Here's how the part is built. I have some questions about the finished solid (model axes, mm). Round coordinates to 2 decimals unless told otherwise and drop trailing zeros. Write each loop counter-clockwise with the first axis right and the second up, starting at its lowest first coordinate (ties: lowest second). Pieces come first, ordered by that corner, then holes. Notation, with made-up numbers: (-16, 29.25) -> (-2, 29.25) arc R15 cw to (-2, 47.25) -> close; hole circle Ø4 at (55, -39). An arc over 180 degrees is marked (long way). Answer in a Markdown table with one row per item.
Autodesk Inventor part; units mm, degrees
ref_plane "YZ Plane" through (0, 0, 0) normal (1, 0, 0) x (0, 1, 0)
ref_plane "XZ Plane" through (0, 0, 0) normal (0, 1, 0) x (-1, 0, 0)
ref_plane "XY Plane" through (0, 0, 0) normal (0, 0, 1) x (1, 0, 0)
sketch "スケッチ1" plane through (0, 0, 0) normal (0, 0, 1) x (1, 0, 0)
  circle A0 centre (0, 0) radius 2
  dimension "d0" = 4
extrude "押し出し1" add sketch "スケッチ1" along normal mid plane 48
chamfer "面取り1" distance 0.1 angle 45 2 edges at (-2, 0, 24) (-2, 0, -24)
sketch "スケッチ2" plane through (0, 0, 0) normal (0, 1, 0) x (-1, 0, 0)
  line L0 (0, 0) -> (3.4806, 0) construction
  line L1 (0, 0) -> (0, -21.75) construction
  circle A0 centre (0, -21.75) radius 0.75
  circle A1 centre (0, 21.75) radius 0.75
  line L2 (2.6688, -21) -> (-4.3603, -21) construction
  dimension "d6" = 1.5
  dimension "d11" = 42
extrude "押し出し2" cut sketch "スケッチ2" along normal through all both and the other way through all
properties part number "COXA_ROLL_SHAFT_D4"
1) I want a section at A-A, the plane x = 0. List the corners of the cut face in (y, z) for me.
Response:
| item | result |
|---|---|
| outline | (-2, -23.9) -> (-1.9, -24) -> (1.9, -24) -> (2, -23.9) -> (2, -22.5) -> (-2, -22.5) -> close; (-2, -21) -> (2, -21) -> (2, 21) -> (-2, 21) -> close; (-2, 22.5) -> (2, 22.5) -> (2, 23.9) -> (1.9, 24) -> (-1.9, 24) -> (-2, 23.9) -> close |
2) I want a section at C-C, the plane z = -21.75. List the corners of the cut face in (x, y) for me.
Response:
| item | result |
|---|---|
| outline | (-0.75, -1.85) -> (-0.75, 1.85) arc R2 ccw to start; (0.75, -1.85) arc R2 ccw to (0.75, 1.85) -> close |
3) I need wall thicknesses on line 1 (Z direction, x = 0, y = 1.2); line 2 (X direction, y = 0.2, z = -21.75); line 3 (X direction, y = -0.1, z = -12). Which ranges of each line are inside material? Lowest first, please. Write a range as [from, to].
Response:
| item | result |
|---|---|
| line 1 | z = [-24, -22.5], [-21, 21], [22.5, 24] |
| line 2 | x = [-1.99, -0.75], [0.75, 1.99] |
| line 3 | x = [-2, 2] |
4) I want a section at B-B, the plane y = 0. List the corners of the cut face in (x, z) for me, and give its area (3 significant figures).
Response:
| item | result |
|---|---|
| outline | (-2, -23.9) -> (-1.9, -24) -> (1.9, -24) -> (2, -23.9) -> (2, 23.9) -> (1.9, 24) -> (-1.9, 24) -> (-2, 23.9) -> close; hole circle Ø1.5 at (0, -21.75); hole circle Ø1.5 at (0, 21.75) |
| area | 188 mm^2 |
5) I want a section at D-D, the plane z = -4.5. List the corners of the cut face in (x, y) for me, and give its area (3 significant figures).
Response:
| item | result |
|---|---|
| outline | circle Ø4 at (0, 0) |
| area | 12.6 mm^2 |
6) We'd pull the mould along Z, two halves only. Please class faces 1 (the face through (0, 0, -24)), 2 (the face through (0, 0, 24)), 3 (the face through (0, 0, -21)): +Z half, -Z half, draft (parallel to the pull), parting line (faces both ways), or undercut.
Response:
| item | result |
|---|---|
| face 1 | -Z half |
| face 2 | +Z half |
| face 3 | undercut |
7) For pin 1 (1 mm diameter, centred on x = 1.5, z = -2.5, fed in from +Y), with a flat end and sliding along its axis, tell me the tip position at first contact or that it passes through.
Response:
| item | result |
|---|---|
| pin 1 | stops at y = 1.73 |
